```python
from build123d import *

# Parameters (mm, degrees)
SKETCH4_R                = 5
BOSS_EXTRUDE1_DEPTH      = 9
SKETCH5_R                = 5.5
BOSS_EXTRUDE2_DEPTH      = 3.5
BOSS_EXTRUDE3_START      = 14.8125
SKETCH6_R                = 5.5
BOSS_EXTRUDE3_DEPTH      = 14.8125
SKETCH7_R                = 4
CUT_EXTRUDE1_DEPTH       = 7
BOSS_EXTRUDE4_DEPTH      = 2
BOSS_EXTRUDE5_DEPTH      = 5.5
BOSS_EXTRUDE5_DEPTH_BACK = 5.5
SKETCH10_R               = 0.5


with BuildPart() as part:
    # Sketch4 → Boss-Extrude1 (new body)
    with BuildSketch(Plane(origin=(0, 0, 0), x_dir=(1, 0, 0), z_dir=(0, 1, 0))):
        with Locations(Location((0, 0, 0), (0, 0, 270))):
            Circle(SKETCH4_R)
    extrude(amount=BOSS_EXTRUDE1_DEPTH)

    # Sketch5 → Boss-Extrude2 (add, symmetric)
    with BuildSketch(Plane(origin=(0, 4.5, 0), x_dir=(1, 0, 0), z_dir=(0, 1, 0))):
        with Locations(Location((0, 0, 0), (0, 0, 270))):
            Circle(SKETCH5_R)
    extrude(amount=BOSS_EXTRUDE2_DEPTH, both=True)

    # Sketch6 → Boss-Extrude3 (add)
    with BuildSketch(Plane(origin=(0, 9, 0), x_dir=(1, 0, 0), z_dir=(0, 1, 0)).offset(BOSS_EXTRUDE3_START)):
        with Locations(Location((0, 0, 0), (0, 0, 270))):
            Circle(SKETCH6_R)
    extrude(amount=-BOSS_EXTRUDE3_DEPTH)

    # Sketch7 → Cut-Extrude1 (cut)
    with BuildSketch(Plane.XZ):
        with Locations(Location((0, 0, 0), (0, 0, 270))):
            Circle(SKETCH7_R)
    extrude(amount=-CUT_EXTRUDE1_DEPTH, mode=Mode.SUBTRACT)

    # Sketch8 → Boss-Extrude4 (add, symmetric)
    with BuildSketch(Plane.XY):
        with BuildLine():
            Line((-2, 23.8125), (2, 23.8125))
            Line((2, 23.8125), (2, 28.575))
            ThreePointArc((2, 28.575), (0, 30.575), (-2, 28.575))
            Line((-2, 28.575), (-2, 23.8125))
        make_face()
    extrude(amount=BOSS_EXTRUDE4_DEPTH, both=True)

    # Sketch10 → Boss-Extrude5 (add, two sides: drawn at the far end of the back side and taken through both)
    with BuildSketch(Plane.XY.offset(-BOSS_EXTRUDE5_DEPTH_BACK)):
        with Locations((0, 28.575)):
            Circle(SKETCH10_R)
    extrude(amount=BOSS_EXTRUDE5_DEPTH + BOSS_EXTRUDE5_DEPTH_BACK)


solid = part.part
```
Geometry: final body of the model. Coordinates: model frame, mm. A direction names the side the tool comes from. Round coordinates to 2 decimals unless told otherwise and drop trailing zeros. Write each loop counter-clockwise with the first axis right and the second up, starting at its lowest first coordinate (ties: lowest second). Pieces come first, ordered by that corner, then holes. Notation, with made-up numbers: M 12.5,32 L 26.5,32 A32 cw 26.5,58 Z; hole C 12.5,-20 d5. An arc over 180 degrees is marked long. Answer in a Markdown table with one row per item. Add a question column.
(1) Cut plane C-C, the plane y = 7.5. Return the cut outline in (x, z).
(2) Reachability of faces 1 (the face through (-3.905, 3.451, 0.867)), 2 (the face through (2, 26, 0)), 3 (the face through (-4.9, 8, 1.6)), 4 (the face through (-0.108, 28.087, -3.774)), 5 (the face through (-0.108, 28.087, 3.726)) from +Z, -Z, +X, -X, +Y, -Y: full face, straight path, thin tool, end or side. Return the list, or none.
(3) Cut plane D-D, the plane z = 0. Return the cut outline in (x, y) (1 decimal), then the cut area to 3 significant figures.
(4) Contact query for flat-ended pins moving along their axis: pin 1 (6.5 mm diameter, centred on x = 0, z = 0, fed in from -Y); pin 2 (4 mm diameter, centred on y = 19.5, z = 3, fed in from +X); pin 3 (1 mm diameter, centred on x = 1, y = 22.5, fed in from -Z). Output: stop coordinate, or through.
(5) Ray query, L1, parallel to X at y = 5, z = 0; L2, parallel to Y at x = -1.25, z = 4.5; L3, parallel to Y at x = 3, z = -4.5. Return the intervals inside material, ascending.
(6) Cut plane A-A, the plane z = -3. Return the cut outline in (x, y) (1 decimal).
(7) Draft query along Y for faces 6 (the face through (0, 7, 0)), 7 (the face through (-2, 26, 0)), 8 (the face through (0, 27, 2)). Return one class per face: pulls with the +Y half, pulls with the -Y half, needs draft (parallel to the pull), parting line crosses it, or undercut.
Established:
| question | item | result |
|---|---|---|
| 1 | outline | C 0,0 d11 |
| 2 | face 1 | -Y |
| 2 | face 2 | +Z, -Z, +X, +Y |
| 2 | face 3 | none |
| 2 | face 4 | -Z |
| 2 | face 5 | +Z |
| 3 | outline | M -5.5,1 L -5,1 L -5,0 L -4,0 L -4,7 L 4,7 L 4,0 L 5,0 L 5,1 L 5.5,1 L 5.5,8 L 5,8 L 5,9 L 5.5,9 L 5.5,23.8 L 2,23.8 L 2,28.6 A2 ccw -2,28.6 L -2,23.8 L -5.5,23.8 L -5.5,9 L -5,9 L -5,8 L -5.5,8 Z |
| 3 | area | 229 mm² |
| 4 | pin 1 | y = 7 |
| 4 | pin 2 | x = 5.41 |
| 4 | pin 3 | z = -5.48 |
| 5 | L1 | -5.5 to -4, 4 to 5.5 |
| 5 | L2 | 0 to 23.81 |
| 5 | L3 | 1 to 8, 9 to 23.81 |
| 6 | outline | M -4.6,1 L -4,1 L -4,0 L -2.6,0 L -2.6,7 L 2.6,7 L 2.6,0 L 4,0 L 4,1 L 4.6,1 L 4.6,8 L 4,8 L 4,9 L 4.6,9 L 4.6,23.8 L -4.6,23.8 L -4.6,9 L -4,9 L -4,8 L -4.6,8 Z; C 0,28.6 d1 |
| 7 | face 6 | pulls with the -Y half |
| 7 | face 7 | needs draft |
| 7 | face 8 | undercut |
